Check sheet for the modelled part. Datum: model origin and axes. Units: mm. A direction names the side the tool comes from. Round coordinates to 2 decimals unless told otherwise and drop trailing zeros. Loops run counter-clockwise (first coordinate to the right, second up) from the corner with the lowest first, then second, coordinate; pieces in that order, holes last. Notation, with made-up numbers: (56, -28) -> (89, -28) arc R28 ccw to (89, -9) -> close; hole circle Ø7 at (67.5, 57.25). An arc over 180 degrees is marked (long way). Use one line per item in the form item = value. Start each with the question number.
(1) Sectioned sample at D-D (z = 0.9). State how many separate pieces and enclosed holes the cut face has, and give its area (3 significant figures).
(2) Sectioned sample at A-A (x = 15). Record the cut outline in (y, z), and give its area (3 significant figures).
(3) Draft check along X on faces 3 (the flat face through (20.624, 13, 1)), 4 (the flat face through (-3.131, 17.218, 0.74)), 5 (the flat face through (60.01, 32.84, 0.74)). Enter one of: released by +X, released by -X, zero draft, split by the parting line, or undercut.
(4) Sectioned sample at C-C (y = 10). Record the cut outline in (x, z), and give its area (3 significant figures).
(5) Material ranges on probe 1 along X at (y, z) = (25, 1.4); probe 2 along Y at (x, z) = (6, 0.8); probe 3 along X at (y, z) = (10.5, 1.4), recorded low to high. Write a range as [from, to].
(6) Set-up check for faces 1 (the cylindrical face through (-2.663, 37.993, 0.74)), 2 (the flat face through (19, 10.824, 1)): record each of +Z, -Z, +X, -X, +Y, -Y from which the full face is reachable in a straight line by a thin tool's end or side.
(7) Go/stop test with a flat-tipped pin: pin 1 (5.5 mm diameter, centred on x = 38.2, y = 28.83, fed in from +Z). Record where the tip stops, or that it passes through.
(8) Sectioned sample at B-B (y = 23). Record the cut outline in (x, z).
from build123d import *

# Parameters (mm, degrees)
MODEL_R         = 1
MODEL_W         = 13.99947
MODEL_H         = 13.99944
MODEL_W_2       = 2.54
MODEL_H_2       = 3.556
MODEL_W_3       = 13.9994
MODEL_W_4       = 13.9993
MODEL_H_3       = 13.9993
MODEL_R_2       = 2.032
MODEL_R_3       = 3.048
EXTRUDE_1_DEPTH = 1.5


with BuildPart() as part:
    # Model → 凸台-拉伸1 (new body)
    with BuildSketch(Plane.XY):
        with BuildLine():
            Line((58.325971896, 38.37894176), (-0.993511809, 38.37894176))
            ThreePointArc((-0.993511809, 38.37894176), (-2.684760262, 37.982445858), (-4.023562246, 36.875585623))
            ThreePointArc((-4.023562246, 36.875585623), (-4.429985557, 35.602098535), (-3.943386617, 34.357040005))
            Line((-3.943386617, 34.357040005), (-1.350000064, 31.36000149))
            Line((-1.350000064, 31.36000149), (-1.353515518, 25.280051374))
            Line((-1.353515518, 25.280051374), (-4.853428588, 21.752613865))
            Line((-4.853428588, 21.752613865), (-4.853710523, 19.020120221))
            Line((-4.853710523, 19.020120221), (-1.359258514, 15.363920359))
            Line((-1.359258514, 15.363920359), (-1.362991715, 8.917997305))
            Line((-1.362991715, 8.917997305), (-4.9049154, 4.538497879))
            Line((-4.9049154, 4.538497879), (-4.9049154, 3.15597541))
            Line((-4.9049154, 3.15597541), (-4.883883595, 2.639206616))
            Line((-4.883883595, 2.639206616), (-4.813264805, 2.011073476))
            Line((-4.813264805, 2.011073476), (-4.687062167, 1.387481119))
            Line((-4.687062167, 1.387481119), (-4.516803943, 0.776764684))
            Line((-4.516803943, 0.776764684), (-4.295659415, 0.187060206))
            Line((-4.295659415, 0.187060206), (-4.03681533, -0.378036856))
            Line((-4.03681533, -0.378036856), (-3.730362364, -0.921623746))
            Line((-3.730362364, -0.921623746), (-3.390574278, -1.434889052))
            Line((-3.390574278, -1.434889052), (-2.992281832, -1.942165148))
            Line((-2.992281832, -1.942165148), (-2.558331876, -2.409802006))
            Line((-2.558331876, -2.409802006), (-2.102251702, -2.829663369))
            Line((-2.102251702, -2.829663369), (-1.614610519, -3.215411153))
            Line((-1.614610519, -3.215411153), (-1.088890304, -3.567123565))
            Line((-1.088890304, -3.567123565), (-0.532800957, -3.878547051))
            Line((-0.532800957, -3.878547051), (0.038326794, -4.140153507))
            Line((0.038326794, -4.140153507), (0.615600502, -4.353028424))
            Line((0.615600502, -4.353028424), (1.223529929, -4.526191258))
            Line((1.223529929, -4.526191258), (1.847223482, -4.64943937))
            Line((1.847223482, -4.64943937), (2.464503115, -4.722060038))
            Line((2.464503115, -4.722060038), (2.992774524, -4.743685))
            Line((2.992774524, -4.743685), (54.34686609, -4.743685))
            Line((54.34686609, -4.743685), (54.87843401, -4.722059086))
            Line((54.87843401, -4.722059086), (55.492240411, -4.649391053))
            Line((55.492240411, -4.649391053), (56.11599848, -4.526806688))
            Line((56.11599848, -4.526806688), (56.726168878, -4.352867841))
            Line((56.726168878, -4.352867841), (57.302144081, -4.140491025))
            Line((57.302144081, -4.140491025), (57.880206411, -3.875955859))
            Line((57.880206411, -3.875955859), (58.434482529, -3.563431063))
            Line((58.434482529, -3.563431063), (58.947571314, -3.220379587))
            Line((58.947571314, -3.220379587), (59.445938304, -2.8287768))
            Line((59.445938304, -2.8287768), (59.905767444, -2.401934126))
            Line((59.905767444, -2.401934126), (60.332973054, -1.941418241))
            Line((60.332973054, -1.941418241), (60.721224007, -1.446690794))
            Line((60.721224007, -1.446690794), (61.064717919, -0.934798534))
            Line((61.064717919, -0.934798534), (61.379380282, -0.376374826))
            Line((61.379380282, -0.376374826), (61.644240363, 0.202684675))
            Line((61.644240363, 0.202684675), (61.855333273, 0.776565869))
            Line((61.855333273, 0.776565869), (62.029241049, 1.384922025))
            Line((62.029241049, 1.384922025), (62.152356641, 2.011350393))
            Line((62.152356641, 2.011350393), (62.226202972, 2.636734827))
            Line((62.226202972, 2.636734827), (62.245297192, 3.166071528))
            Line((62.245297192, 3.166071528), (58.745412398, 6.86443549))
            Line((58.745412398, 6.86443549), (58.745666056, 15.007268129))
            Line((58.745666056, 15.007268129), (62.245579127, 18.534705638))
            Line((62.245579127, 18.534705638), (62.245861062, 21.267199282))
            Line((62.245861062, 21.267199282), (58.745975132, 24.929084585))
            Line((58.745975132, 24.929084585), (58.746175407, 31.358234918))
            Line((58.746175407, 31.358234918), (61.304557204, 34.355344918))
            ThreePointArc((61.304557204, 34.355344918), (61.782522432, 35.594711806), (61.37863268, 36.860158015))
            ThreePointArc((61.37863268, 36.860158015), (60.030777011, 37.978272972), (58.325971896, 38.37894176))
        make_face()
        with Locations((8.744501265, -2.189788582)):
            Circle(MODEL_R, mode=Mode.SUBTRACT)
        with Locations((9.620765, 9.78198)):
            Rectangle(MODEL_W, MODEL_H, mode=Mode.SUBTRACT)
        with Locations((19.353985322, 12.60229784)):
            Rectangle(MODEL_W_2, MODEL_H_2, mode=Mode.SUBTRACT)
        with Locations((48.744501265, -2.189788582)):
            Circle(MODEL_R, mode=Mode.SUBTRACT)
        with Locations((28.6707, 9.78198)):
            Rectangle(MODEL_W_3, MODEL_H, mode=Mode.SUBTRACT)
        with Locations((47.72075, 9.78198)):
            Rectangle(MODEL_W_4, MODEL_H, mode=Mode.SUBTRACT)
        with Locations((-2.255498735, 20.010211418)):
            Circle(MODEL_R, mode=Mode.SUBTRACT)
        with Locations((9.620765, 28.83195)):
            Rectangle(MODEL_W, MODEL_H_3, mode=Mode.SUBTRACT)
        with Locations((-1.568763471, 34.380826193)):
            Circle(MODEL_R, mode=Mode.SUBTRACT)
        with Locations((19.1458, 28.832)):
            Circle(MODEL_R_2, mode=Mode.SUBTRACT)
        with Locations((59.944501265, 20.010211418)):
            Circle(MODEL_R, mode=Mode.SUBTRACT)
        with Locations((28.6708, 28.832)):
            Circle(MODEL_R_3, mode=Mode.SUBTRACT)
        with Locations((38.1958, 28.832)):
            Circle(MODEL_R_2, mode=Mode.SUBTRACT)
        with Locations((47.72075, 28.83195)):
            Rectangle(MODEL_W_4, MODEL_H_3, mode=Mode.SUBTRACT)
        with Locations((58.931236529, 34.380826193)):
            Circle(MODEL_R, mode=Mode.SUBTRACT)
    extrude(amount=EXTRUDE_1_DEPTH)


solid = part.part
Checks:
q1.separate_pieces = 1
q1.enclosed_holes = 15
q1.area = 1,650 mm2
q2.outline = (-4.74, 0) -> (2.78, 0) -> (2.78, 1.5) -> (-4.74, 1.5) -> close; (16.78, 0) -> (21.83, 0) -> (21.83, 1.5) -> (16.78, 1.5) -> close; (35.83, 0) -> (38.38, 0) -> (38.38, 1.5) -> (35.83, 1.5) -> close
q2.area = 22.7 mm2
q3.face_3 = undercut
q3.face_4 = released by -X
q3.face_5 = released by +X
q4.outline = (-1.36, 0) -> (2.62, 0) -> (2.62, 1.5) -> (-1.36, 1.5) -> close; (16.62, 0) -> (21.67, 0) -> (21.67, 1.5) -> (16.62, 1.5) -> close; (35.67, 0) -> (40.72, 0) -> (40.72, 1.5) -> (35.67, 1.5) -> close; (54.72, 0) -> (58.75, 0) -> (58.75, 1.5) -> (54.72, 1.5) -> close
q4.area = 27.2 mm2
q5.probe_1 = [-1.63, 2.62], [16.62, 40.72], [54.72, 58.75]
q5.probe_2 = [-4.74, 2.78], [16.78, 21.83], [35.83, 38.38]
q5.probe_3 = [-1.36, 2.62], [16.62, 21.67], [35.67, 40.72], [54.72, 58.75]
q6.face_1 = +Z, -Z, -X, +Y
q6.face_2 = +Z, -Z
q7.pin_1 = 1.5
q8.outline = (-3.62, 0) -> (2.62, 0) -> (2.62, 1.5) -> (-3.62, 1.5) -> close; (16.62, 0) -> (40.72, 0) -> (40.72, 1.5) -> (16.62, 1.5) -> close; (54.72, 0) -> (60.59, 0) -> (60.59, 1.5) -> (54.72, 1.5) -> close
